Input: dimensioned drawing with shaded views. Units: mm. Origin: part minimum x, y, z. Round coordinates to 2 decimals unless told otherwise and drop trailing zeros. Loops run counter-clockwise (first coordinate to the right, second up) from the corner with the lowest first, then second, coordinate; pieces in that order, holes last. Notation, with made-up numbers: M 43,18.25 L 49,18.25 A11 ccw 49,34.25 Z; hole C 63,-4 d5. An arc over 180 degrees is marked long. One line per item, written item: value.
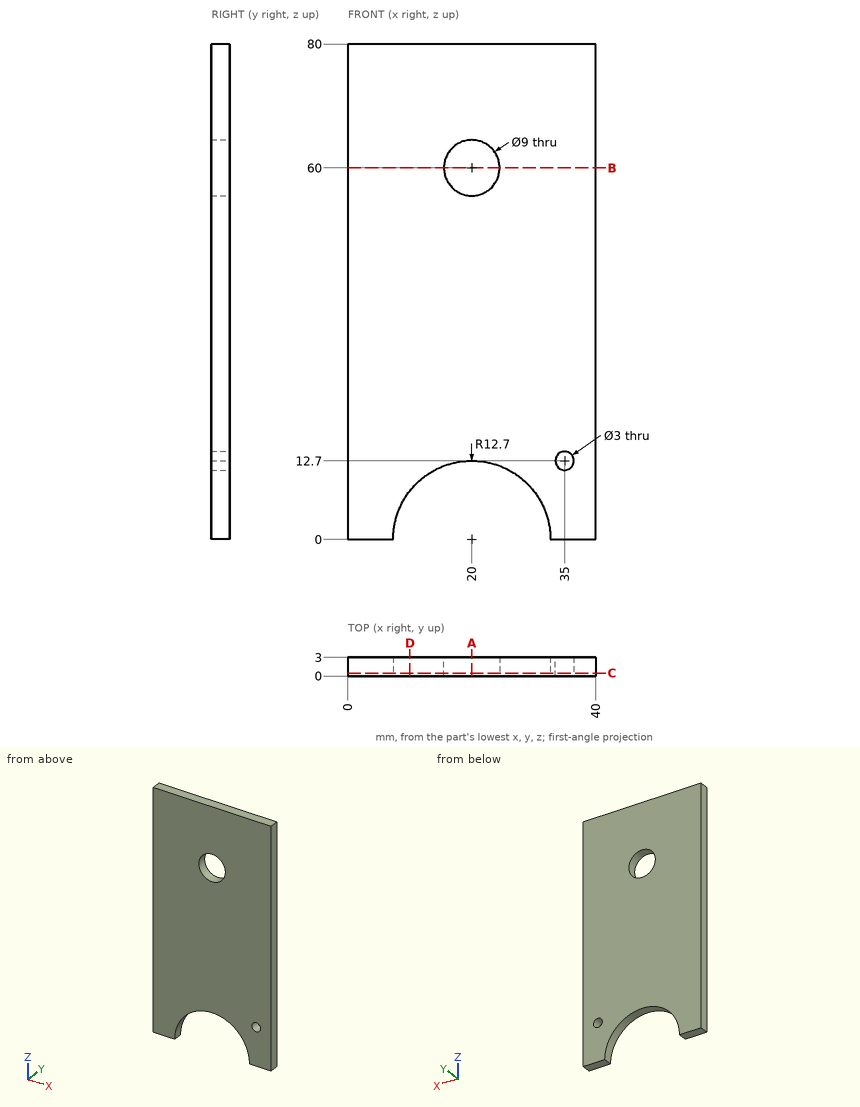
1. Section query A-A (x = 20). Return the cut outline in (y, z), and give its area (3 significant figures).
Report:
outline: M 0,12.7 L 3,12.7 L 3,55.5 L 0,55.5 Z; M 0,64.5 L 3,64.5 L 3,80 L 0,80 Z
area: 175 mm2
2. Section query B-B (z = 60). Return the cut outline in (x, y).
Report:
outline: M 0,0 L 15.5,0 L 15.5,3 L 0,3 Z; M 24.5,0 L 40,0 L 40,3 L 24.5,3 Z
3. Ray query, line 1 (Z direction, x = 20, y = 1.2); line 2 (Z direction, x = 35, y = 1.4); line 3 (X direction, y = 2.05, z = 9). Return the intervals inside material, ascending. Write a range as [from, to].
Report:
line 1: z = [12.7, 55.5], [64.5, 80]
line 2: z = [0, 11.2], [14.2, 80]
line 3: x = [0, 11.04], [28.96, 40]
4. Section query D-D (x = 10). Return the cut outline in (y, z).
Report:
outline: M 0,7.83 L 3,7.83 L 3,80 L 0,80 Z
5. Pin query (flat end, axial travel): pin 1 (1.8 mm diameter, centred on x = 35, z = 12.7, fed in from +Y). Return the tip coordinate at first contact, or that it passes through.
Report:
pin 1: passes through
6. Section query C-C (y = 0.45). Return the cut outline in (x, z).
Report:
outline: M 0,0 L 7.3,0 A12.7 cw 32.7,0 L 40,0 L 40,80 L 0,80 Z; hole C 20,60 d9; hole C 35,12.7 d3
